Read the model definition and answer for the solid it produces. Units are mm, in the model's axes. Face numbers are marked on the shaded views. A direction names the side the tool comes from. Coordinates: 2 decimals unless noted, no trailing zeros. Order: outer loops, then holes, each group sorted by start corner. A loop starts at its lowest first (then second) coordinate and runs counter-clockwise, first axis right, second up.
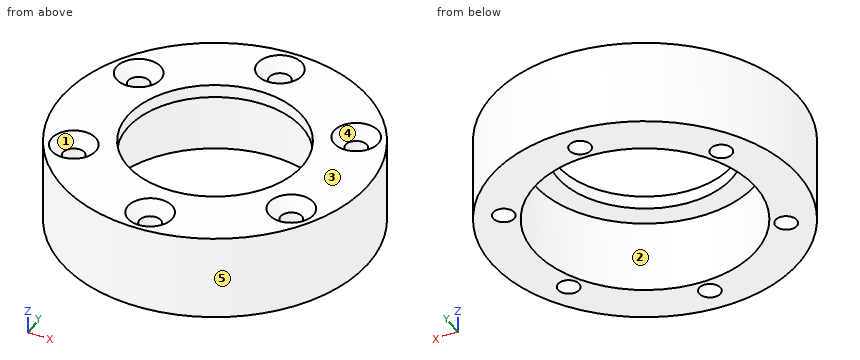
```python
from build123d import *

# Parameters (mm, degrees)
SKETCH1_R                                       = 32.5
BOSS_EXTRUDE1_DEPTH                             = 18
CSK_FOR_M4_FLAT_HEAD_MACHINE_SCREW1_D           = 4.5
CSK_FOR_M4_FLAT_HEAD_MACHINE_SCREW1_CSINK_D     = 9.4
CSK_FOR_M4_FLAT_HEAD_MACHINE_SCREW1_CSINK_ANGLE = 90
CIRPATTERN1_COUNT                               = 6
SKETCH4_R                                       = 18.5
CUT_EXTRUDE1_DEPTH                              = 30
SKETCH5_R                                       = 23.5
CUT_EXTRUDE2_DEPTH                              = 15.25


with BuildPart() as part:
    # Sketch1 → Boss-Extrude1 (new body)
    with BuildSketch(Plane.XY):
        Circle(SKETCH1_R)
    extrude(amount=BOSS_EXTRUDE1_DEPTH)

    # CSK for M4 Flat Head Machine Screw1 (through all)
    with Locations(Plane.XY.offset(18)):
        with Locations((0, 26.7)):
            csk_for_m4_flat_head_machine_screw1 = CounterSinkHole(CSK_FOR_M4_FLAT_HEAD_MACHINE_SCREW1_D / 2, CSK_FOR_M4_FLAT_HEAD_MACHINE_SCREW1_CSINK_D / 2, counter_sink_angle=CSK_FOR_M4_FLAT_HEAD_MACHINE_SCREW1_CSINK_ANGLE)

    # CirPattern1: CSK for M4 Flat Head Machine Screw1 ×6 about axis
    cirpattern1_axis = Axis((0, 0, 0), (0, 0, 1))
    for i in range(1, CIRPATTERN1_COUNT):
        add(csk_for_m4_flat_head_machine_screw1.rotate(cirpattern1_axis, i * 360 / CIRPATTERN1_COUNT), mode=Mode.SUBTRACT)

    # Sketch4 → Cut-Extrude1 (cut)
    with BuildSketch(Plane(origin=(0, 0, 0), x_dir=(-1, 0, 0), z_dir=(0, 0, -1))):
        Circle(SKETCH4_R)
    extrude(amount=-CUT_EXTRUDE1_DEPTH, mode=Mode.SUBTRACT)

    # Sketch5 → Cut-Extrude2 (cut)
    with BuildSketch(Plane(origin=(0, 0, 0), x_dir=(-1, 0, 0), z_dir=(0, 0, -1))):
        Circle(SKETCH5_R)
    extrude(amount=-CUT_EXTRUDE2_DEPTH, mode=Mode.SUBTRACT)


solid = part.part
```
1) A cutting plane is placed at B-B, the plane x = 0. Determine the outline of the cut face in (y, z).
A:
outline: (-32.5, 0) - (-28.95, 0) - (-28.95, 15.55) - (-31.4, 18) - (-32.5, 18) - close; (-24.45, 0) - (-23.5, 0) - (-23.5, 15.25) - (-18.5, 15.25) - (-18.5, 18) - (-22, 18) - (-24.45, 15.55) - close; (18.5, 15.25) - (23.5, 15.25) - (23.5, 0) - (24.45, 0) - (24.45, 15.55) - (22, 18) - (18.5, 18) - close; (28.95, 0) - (32.5, 0) - (32.5, 18) - (31.4, 18) - (28.95, 15.55) - close
2) A cutting plane is placed at C-C, the plane y = 13.35. Determine the outline of the cut face in (x, z), and give its area (3 significant figures).
A:
outline: (-29.63, 0) - (-25.37, 0) - (-25.37, 15.55) - (-27.82, 18) - (-29.63, 18) - close; (-20.87, 0) - (-19.34, 0) - (-19.34, 15.25) - (-12.81, 15.25) - (-12.81, 18) - (-18.42, 18) - (-20.87, 15.55) - close; (12.81, 15.25) - (19.34, 15.25) - (19.34, 0) - (20.87, 0) - (20.87, 15.55) - (18.42, 18) - (12.81, 18) - close; (25.37, 0) - (29.63, 0) - (29.63, 18) - (27.82, 18) - (25.37, 15.55) - close
area: 232 mm2
3) Which of the six approach directions +Z, -Z, +X, -X, +Y, -Y give full straight-line access (tool end or side, diameter ignored) to the marked faces 1 and 2?
A:
face 1: +Z
face 2: -Z
4) Determine the mould class of the marked faces 3, 4 and 5 for opening direction X: pulls with the +X half, pulls with the -X half, needs draft (parallel to the pull), parting line crosses it, or undercut.
A:
face 3: needs draft
face 4: undercut
face 5: parting line crosses it
5) A cutting plane is placed at D-D, the plane z = 14.5. Determine the outline of the cut face in (x, y), and give its area (3 significant figures).
A:
outline: circle Ø65 at (0, 0); hole circle Ø4.5 at (-23.12, -13.35); hole circle Ø4.5 at (-23.12, 13.35); hole circle Ø47 at (0, 0); hole circle Ø4.5 at (0, -26.7); hole circle Ø4.5 at (0, 26.7); hole circle Ø4.5 at (23.12, -13.35); hole circle Ø4.5 at (23.12, 13.35)
area: 1,490 mm2
6) A cutting plane is placed at A-A, the plane y = 0. Determine the outline of the cut face in (x, z).
A:
outline: (-32.5, 0) - (-23.5, 0) - (-23.5, 15.25) - (-18.5, 15.25) - (-18.5, 18) - (-32.5, 18) - close; (18.5, 15.25) - (23.5, 15.25) - (23.5, 0) - (32.5, 0) - (32.5, 18) - (18.5, 18) - close
7) Straight lines are drawn through the part: line 1 (Y direction, x = 0, z = 12.5); line 2 (X direction, y = -14, z = 15.75); line 3 (X direction, y = 13.5, z = 2.25). For each, find the intervals that lie inside material, in ascending order.
A:
line 1: y = -32.5 to -28.95, -24.45 to -23.5, 23.5 to 24.45, 28.95 to 32.5
line 2: x = -29.33 to -25.49, -20.76 to -12.09, 12.09 to 20.76, 25.49 to 29.33
line 3: x = -29.56 to -25.37, -20.88 to -19.24, 19.24 to 20.88, 25.37 to 29.56
8) Flat-ended cylindrical pins translate along their axes: pin 1 Ø3 at (y, z) = (17.5, 6) entering from +X; pin 2 Ø4 at (x, y) = (0, -26.7) entering from +Z; pin 3 Ø3 at (y, z) = (-21, 6) entering from -X; pin 4 Ø4 at (x, z) = (-17.5, 13.5) entering from +Y. Find the tip coordinate at first contact, or state that the pin passes through.
A:
pin 1: stops at x = 28.29
pin 2: passes through
pin 3: stops at x = -26
pin 4: stops at y = 28.57
